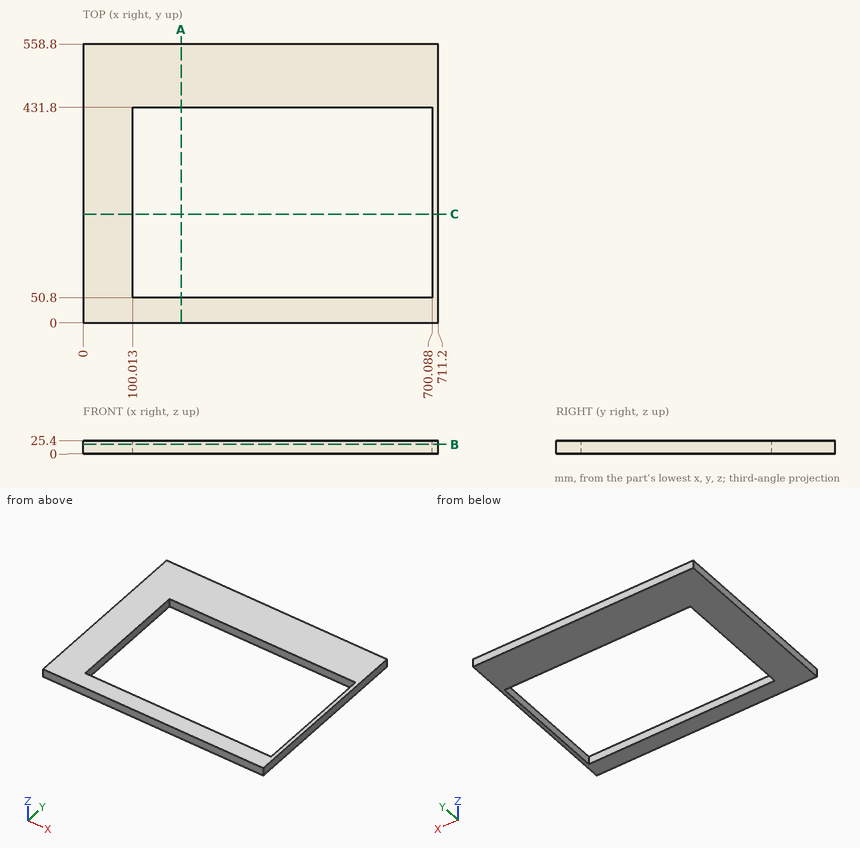
Input: dimensioned drawing with shaded views. Units: mm. Origin: part minimum x, y, z. Coordinates: 2 decimals unless noted, no trailing zeros. Loops run counter-clockwise (first coordinate to the right, second up) from the corner with the lowest first, then second, coordinate; pieces in that order, holes last. Notation, with made-up numbers: M 30.25,-12 L 72.25,-12 A20 cw 72.25,7 Z; hole C 64,71 d4. An arc over 180 degrees is marked long. Use a Markdown table: item, result. Add a question column.
1) Section C-C, the plane y = 218. Return the cut outline in (x, z).
2) Line query: L1, parallel to Y at x = 478, z = 21; L2, parallel to X at y = 78, z = 19.75. Output: solid intervals per line, ascending. Write a range as from..to.
3) Section B-B, the plane z = 18.5. Return the cut outline in (x, y), plus the area to 3 significant figures.
4) Section A-A, the plane x = 196.5. Return the cut outline in (y, z), plus the area to 3 significant figures.
Answer below:
| question | item | result |
|---|---|---|
| 1 | outline | M 0,0 L 100.01,0 L 100.01,25.4 L 0,25.4 Z; M 700.09,0 L 711.2,0 L 711.2,25.4 L 700.09,25.4 Z |
| 2 | L1 | 0..50.8, 431.8..558.8 |
| 2 | L2 | 0..100.01, 700.09..711.2 |
| 3 | outline | M 0,0 L 711.2,0 L 711.2,558.8 L 0,558.8 Z; hole M 100.01,50.8 L 700.09,50.8 L 700.09,431.8 L 100.01,431.8 Z |
| 3 | area | 169,000 mm2 |
| 4 | outline | M 0,0 L 50.8,0 L 50.8,25.4 L 0,25.4 Z; M 431.8,0 L 558.8,0 L 558.8,25.4 L 431.8,25.4 Z |
| 4 | area | 4,520 mm2 |
